Part model, mm, in its own coordinate system. Face numbers are marked on the shaded views. A direction names the side the tool comes from. Coordinates: 2 decimals unless noted, no trailing zeros. Loops run counter-clockwise (first coordinate to the right, second up) from the corner with the lowest first, then second, coordinate; pieces in that order, holes last. Notation, with made-up numbers: (76.5, 83.5) - (93.5, 83.5) arc R27 cw to (93.5, 99.5) - close; hole circle Ø10 at (85.5, 34). An arc over 180 degrees is marked (long way). Answer as CSV lines item,"result".
from build123d import *

# Parameters (mm, degrees)
ESQUISSE2_W                                        = 38
ESQUISSE2_H                                        = 22
BOSS_EXTRU_1_DEPTH                                 = 20
CHAMBRAGE_POUR_VIS_T_TE_HEXAGONALE_M31_D           = 3.4
CHAMBRAGE_POUR_VIS_T_TE_HEXAGONALE_M31_CBORE_D     = 6.5
CHAMBRAGE_POUR_VIS_T_TE_HEXAGONALE_M31_CBORE_DEPTH = 3.4
CONG_1_R                                           = 1


with BuildPart() as part:
    # Esquisse2 → Boss.-Extru.1 (new body)
    with BuildSketch(Plane(origin=(0, 0, 0), x_dir=(1, 0, 0), z_dir=(0, 1, 0))):
        Rectangle(ESQUISSE2_W, ESQUISSE2_H)
    extrude(amount=BOSS_EXTRU_1_DEPTH)

    # Chambrage pour vis à tête hexagonale M31 (through all)
    with Locations(Plane(origin=(0, 20, 0), x_dir=(1, 0, 0), z_dir=(0, 1, 0))):
        with Locations((-9, 0), (9, 0)):
            CounterBoreHole(CHAMBRAGE_POUR_VIS_T_TE_HEXAGONALE_M31_D / 2, CHAMBRAGE_POUR_VIS_T_TE_HEXAGONALE_M31_CBORE_D / 2, CHAMBRAGE_POUR_VIS_T_TE_HEXAGONALE_M31_CBORE_DEPTH)

    # Congé1
    cong_1_edges = [part.edges().sort_by_distance(p)[0] for p in [
        (0, 20, -11),
        (0, 20, 11),
    ]]
    fillet(cong_1_edges, radius=CONG_1_R)


solid = part.part
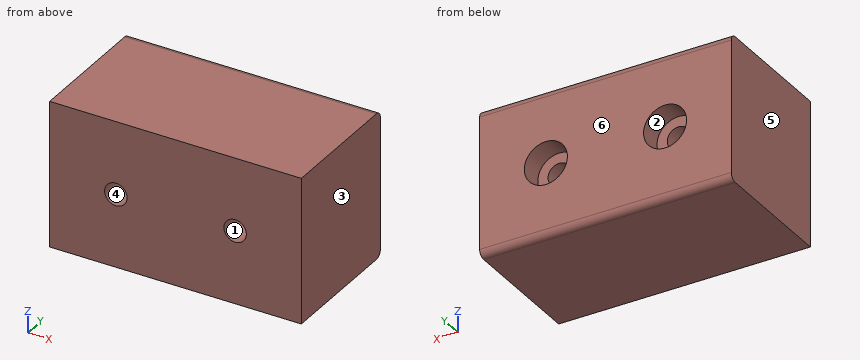
Q1. Flat gauge pin, fed straight in: pin 1 (3 mm diameter, centred on x = -7.5, z = -0.5, fed in from +Y). Where does the tip first touch, or does it go through?
Results:
pin 1,"stops at y = 16.6"
Q2. Wall check: L1, parallel to Z at x = -9, y = 17.7; L2, parallel to Z at x = 9, y = 14.5; L3, parallel to X at y = 10.25, z = 0.75. Give the ranges that are in metal, low to high.
Results:
L1,"z = -11 to -3.25, 3.25 to 11"
L2,"z = -11 to -1.7, 1.7 to 11"
L3,"x = -19 to -10.53, -7.47 to 7.47, 10.53 to 19"
Q3. Saw through at A-A (x = 9). Give the cut face in (y, z).
Results:
outline,"(0, -11) - (19, -11) arc R1 ccw to (20, -10) - (20, -3.25) - (16.6, -3.25) - (16.6, -1.7) - (0, -1.7) - close; (0, 1.7) - (16.6, 1.7) - (16.6, 3.25) - (20, 3.25) - (20, 10) arc R1 ccw to (19, 11) - (0, 11) - close"
Q4. Which spindle directions (+Z, -Z, +X, -X, +Y, -Y) get a long thin tool onto all of the face, cutting with end or side? Do the marked faces 1 and 2. Say none if no direction does.
Results:
face 1,"+Y, -Y"
face 2,"+Y"
Q5. Saw through at B-B (z = 0). Give the cut face in (x, y).
Results:
outline,"(-19, 0) - (-10.7, 0) - (-10.7, 16.6) - (-12.25, 16.6) - (-12.25, 20) - (-19, 20) - close; (-7.3, 0) - (7.3, 0) - (7.3, 16.6) - (5.75, 16.6) - (5.75, 20) - (-5.75, 20) - (-5.75, 16.6) - (-7.3, 16.6) - close; (10.7, 0) - (19, 0) - (19, 20) - (12.25, 20) - (12.25, 16.6) - (10.7, 16.6) - close"
Q6. Saw through at C-C (y = 15). Give the cut face in (x, z).
Results:
outline,"(-19, -11) - (19, -11) - (19, 11) - (-19, 11) - close; hole circle Ø3.4 at (-9, 0); hole circle Ø3.4 at (9, 0)"
Q7. Saw through at D-D (z = -2.5). Give the cut face in (x, y).
Results:
outline,"(-19, 0) - (19, 0) - (19, 20) - (11.08, 20) - (11.08, 16.6) - (6.92, 16.6) - (6.92, 20) - (-6.92, 20) - (-6.92, 16.6) - (-11.08, 16.6) - (-11.08, 20) - (-19, 20) - close"
Q8. Two-plate mould, pull along X, no slides. Class the marked faces 3, 4, 5 and 6: released by +X, released by -X, zero draft, split by the parting line, or undercut.
Results:
face 3,"released by +X"
face 4,"undercut"
face 5,"released by -X"
face 6,"zero draft"
